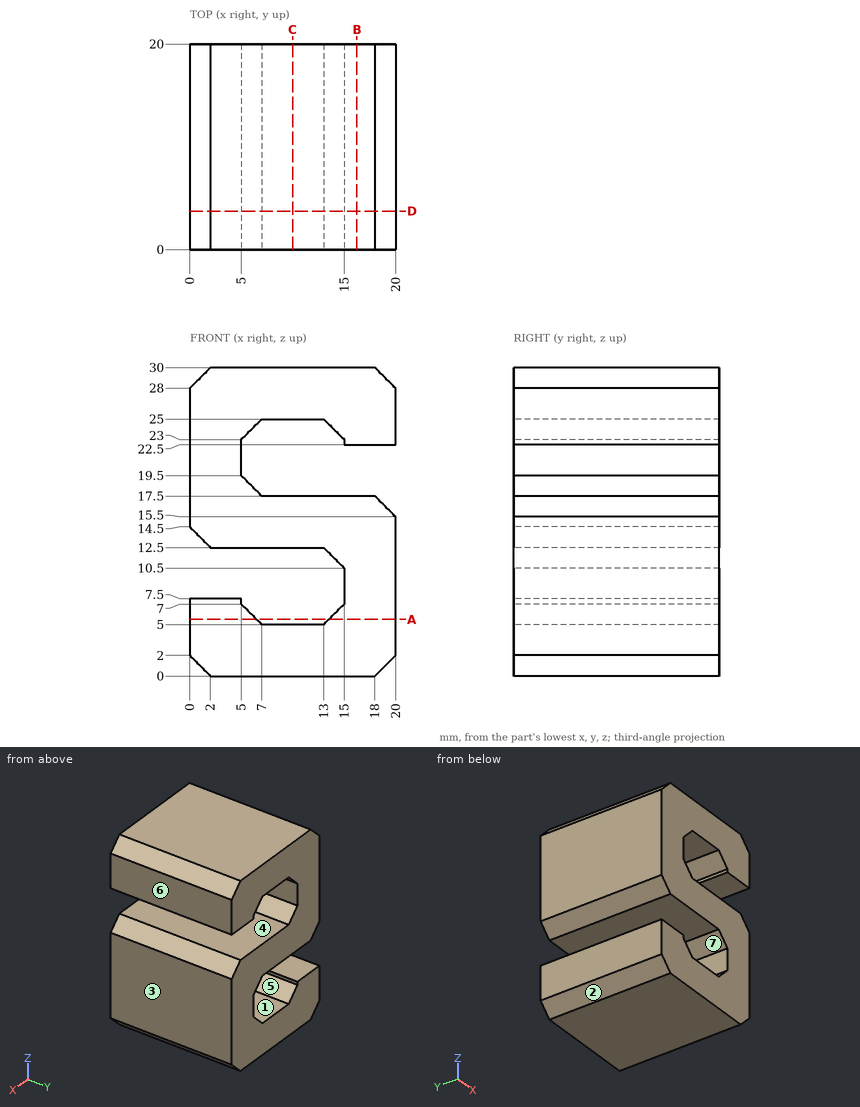
Design review of the part shown in the three views and the two pictorial views. Dimensions are in mm from the part's minimum x, y and z. A direction names the side the tool comes from. Round coordinates to 2 decimals unless told otherwise and drop trailing zeros. Write each loop counter-clockwise with the first axis right and the second up, starting at its lowest first coordinate (ties: lowest second). Pieces come first, ordered by that corner, then holes. Notation, with made-up numbers: M 64.5,-2.75 L 90.5,-2.75 A15 cw 90.5,19.25 Z; hole C 85.5,-9.5 d3. An arc over 180 degrees is marked long. Use a Markdown table: item, result. Add a question column.
Q1. To check wall thickness, follow line 1 (Z direction, x = 8.25, y = 15.75); line 2 (Z direction, x = 17, y = 9.75); line 3 (Z direction, x = 2.75, y = 9.25). State the ranges of each line that lie inside material, in increasing order.
Q2. Machinability: for the marked faces 4, 5, 6 and 7, which of the approach directions +Z, -Z, +X, -X, +Y, -Y give a long, thin tool a straight path to every point of the face, cutting with its end or side? Answer none if there is none.
Q3. Insertion check: pin 1 (1 mm diameter, centred on y = 8.5, z = 13, fed in from -X); pin 2 (1.8 mm diameter, centred on y = 10, z = 9, fed in from -X); pin 3 (2 mm diameter, centred on y = 14, z = 19.5, fed in from +X). Each pin has a flat end and moves straight along its axis. Give the tip position at first contact, or say it passes through.
Q4. We need section B-B, the plane x = 16.25. State the section outline as (y, z) points.
Q5. We need section A-A, the plane z = 5.5. State the section outline as (x, y) points, plus the area to 3 significant figures.
Q6. We need section D-D, the plane y = 3.75. State the section outline as (x, z) points.
Q7. The part is to be moulded in two halves that separate along Z. For the marked faces 1, 2 and 3, say which applies: pulls with the +Z half, pulls with the -Z half, needs draft (parallel to the pull), parting line crosses it, or undercut.
Q8. We need section C-C, the plane x = 10. State the section outline as (y, z) points.
Findings below:
| question | item | result |
|---|---|---|
| 1 | line 1 | z = 0 to 5, 12.5 to 17.5, 25 to 30 |
| 1 | line 2 | z = 0 to 17.5, 22.5 to 30 |
| 1 | line 3 | z = 0 to 7.5, 12.5 to 30 |
| 2 | face 4 | +X, +Y, -Y |
| 2 | face 5 | +Y, -Y |
| 2 | face 6 | +Z, -Z, +X, +Y, -Y |
| 2 | face 7 | -X, +Y, -Y |
| 3 | pin 1 | stops at x = 1 |
| 3 | pin 2 | stops at x = 15 |
| 3 | pin 3 | stops at x = 6 |
| 4 | outline | M 0,0 L 20,0 L 20,17.5 L 0,17.5 Z; M 0,22.5 L 20,22.5 L 20,30 L 0,30 Z |
| 5 | outline | M 0,0 L 6.5,0 L 6.5,20 L 0,20 Z; M 13.5,0 L 20,0 L 20,20 L 13.5,20 Z |
| 5 | area | 260 mm² |
| 6 | outline | M 0,2 L 2,0 L 18,0 L 20,2 L 20,15.5 L 18,17.5 L 7,17.5 L 5,19.5 L 5,23 L 7,25 L 13,25 L 15,23 L 15,22.5 L 20,22.5 L 20,28 L 18,30 L 2,30 L 0,28 L 0,14.5 L 2,12.5 L 13,12.5 L 15,10.5 L 15,7 L 13,5 L 7,5 L 5,7 L 5,7.5 L 0,7.5 Z |
| 7 | face 1 | undercut |
| 7 | face 2 | pulls with the -Z half |
| 7 | face 3 | needs draft |
| 8 | outline | M 0,0 L 20,0 L 20,5 L 0,5 Z; M 0,12.5 L 20,12.5 L 20,17.5 L 0,17.5 Z; M 0,25 L 20,25 L 20,30 L 0,30 Z |
